CAD build for the part. Positions are in the model's coordinates, mm. A direction names the side the tool comes from. Coordinates: 2 decimals unless noted, no trailing zeros. Write each loop counter-clockwise with the first axis right and the second up, starting at its lowest first coordinate (ties: lowest second). Pieces come first, ordered by that corner, then holes. Notation, with made-up numbers: (-23, -11.5) -> (0, -11.5) arc R21 ccw to (0, -2.5) -> close; hole circle Ø6 at (42, 80.5). An arc over 180 degrees is marked (long way). Answer as CSV lines item,"result".
```python
from build123d import *

# Parameters (mm, degrees)
BOSS_EXTRUDE1_DEPTH = 7.75
SKETCH2_R           = 6.125
CUT_EXTRUDE1_DEPTH  = 4.25
CUT_EXTRUDE2_REACH  = 5.5
SKETCH3_R           = 2.125
SKETCH4_R           = 11
BOSS_EXTRUDE2_DEPTH = 20
SKETCH5_R           = 2.25
SKETCH5_R_2         = 4
CUT_EXTRUDE3_DEPTH  = 10
SKETCH6_R           = 2.125
CUT_EXTRUDE4_DEPTH  = 28.75
SKETCH10_R          = 2.75
CUT_EXTRUDE5_DEPTH  = 6


with BuildPart() as part:
    # Sketch1 → Boss-Extrude1 (new body)
    with BuildSketch(Plane.XY):
        with BuildLine():
            ThreePointArc((-12.5, 0), (0, -12.5), (12.5, 0))
            add(Edge.make_bspline(
                [(7.5, 49.5), (7.5, 26.668276539), (12.5, 15.631461909), (12.5, 0)],
                knots=[0, 0, 0, 0, 1, 1, 1, 1], degree=3))
            ThreePointArc((7.5, 49.5), (0, 57), (-7.5, 49.5))
            add(Edge.make_bspline(
                [(-7.5, 49.5), (-7.5, 26.668276539), (-12.5, 15.631461909), (-12.5, 0)],
                knots=[0, 0, 0, 0, 1, 1, 1, 1], degree=3))
        make_face()
    extrude(amount=BOSS_EXTRUDE1_DEPTH)

    # Sketch2 → Cut-Extrude1 (cut)
    with BuildSketch(Plane.XY.offset(7.75)):
        with Locations((0, 49.5)):
            Circle(SKETCH2_R)
    extrude(amount=-CUT_EXTRUDE1_DEPTH, mode=Mode.SUBTRACT)

    # Sketch3 → Cut-Extrude2 (cut, up to next)
    with BuildSketch(Plane.XY.offset(3.5), mode=Mode.PRIVATE) as cut_extrude2_sk1:
        with Locations((0, 49.5)):
            Circle(SKETCH3_R)
    cut_extrude2_tool1 = extrude(cut_extrude2_sk1.sketch, amount=-CUT_EXTRUDE2_REACH, mode=Mode.PRIVATE) & part.part
    add(cut_extrude2_tool1.solids().sort_by_distance((0, 49.5, 3.5))[0], mode=Mode.SUBTRACT)

    # Sketch4 → Boss-Extrude2 (add)
    with BuildSketch(Plane.XY.offset(7.75)):
        Circle(SKETCH4_R)
    extrude(amount=BOSS_EXTRUDE2_DEPTH)

    # Sketch5 → Cut-Extrude3 (cut)
    with BuildSketch(Plane.XY.offset(27.75)):
        with Locations((5.303300859, 5.303300859)):
            Circle(SKETCH5_R)
        with Locations((5.303300859, -5.303300859)):
            Circle(SKETCH5_R)
        with Locations((-5.303300859, -5.303300859)):
            Circle(SKETCH5_R)
        with Locations((-5.303300859, 5.303300859)):
            Circle(SKETCH5_R)
        Circle(SKETCH5_R_2)
    extrude(amount=-CUT_EXTRUDE3_DEPTH, mode=Mode.SUBTRACT)

    # Sketch6 → Cut-Extrude4 (cut, through all)
    with BuildSketch(Plane(origin=(0, 0, 0), x_dir=(-1, 0, 0), z_dir=(0, 0, -1))):
        Circle(SKETCH6_R)
    extrude(amount=-CUT_EXTRUDE4_DEPTH, mode=Mode.SUBTRACT)

    # Sketch10 → Cut-Extrude5 (cut)
    with BuildSketch(Plane(origin=(0, 0, 0), x_dir=(-1, 0, 0), z_dir=(0, 0, -1))):
        Circle(SKETCH10_R)
    extrude(amount=-CUT_EXTRUDE5_DEPTH, mode=Mode.SUBTRACT)


solid = part.part
```
Item 1: Wall check: line 1 (Y direction, x = 0, z = 2.1) (3 decimals); line 2 (Y direction, x = 0, z = 25); line 3 (X direction, y = -5, z = 19). Give the ranges that are in metal, low to high. Write a range as from..to.
Answer below:
line 1,"y = -12.5..-2.75, 2.75..47.375, 51.625..57"
line 2,"y = -11..-4, 4..11"
line 3,"x = -9.8..-7.53, -3.07..3.07, 7.53..9.8"
Item 2: Saw through at A-A on x = 0. Give the cut face in (y, z) (3 decimals), and give its area (3 significant figures).
Answer below:
outline,"(-12.5, 0) -> (-2.75, 0) -> (-2.75, 6) -> (-2.125, 6) -> (-2.125, 17.75) -> (-4, 17.75) -> (-4, 27.75) -> (-11, 27.75) -> (-11, 7.75) -> (-12.5, 7.75) -> close; (2.125, 6) -> (2.75, 6) -> (2.75, 0) -> (47.375, 0) -> (47.375, 3.5) -> (43.375, 3.5) -> (43.375, 7.75) -> (11, 7.75) -> (11, 27.75) -> (4, 27.75) -> (4, 17.75) -> (2.125, 17.75) -> close; (51.625, 0) -> (57, 0) -> (57, 7.75) -> (55.625, 7.75) -> (55.625, 3.5) -> (51.625, 3.5) -> close"
area,"749 mm2"
Item 3: Saw through at B-B on z = 9.75. Give the cut face in (x, y) (3 decimals), and give its area (3 significant figures).
Answer below:
outline,"circle Ø22 at (0, 0); hole circle Ø4.25 at (0, 0)"
area,"366 mm2"
Item 4: Flat gauge pins, fed straight in: pin 1 (2.5 mm diameter, centred on x = 5.3, y = -5.3, fed in from +Z); pin 2 (3 mm diameter, centred on y = 1.5, z = 20.5, fed in from +X); pin 3 (8 mm diameter, centred on y = 32, z = 6, fed in from +X). Where does each tip first touch, or does it go through?
Answer below:
pin 1,"stops at z = 17.75"
pin 2,"stops at x = 11"
pin 3,"stops at x = 9.07"
Item 5: Saw through at C-C on z = 25.5. Give the cut face in (x, y).
Answer below:
outline,"circle Ø22 at (0, 0); hole circle Ø4.5 at (-5.3, -5.3); hole circle Ø4.5 at (-5.3, 5.3); hole circle Ø8 at (0, 0); hole circle Ø4.5 at (5.3, -5.3); hole circle Ø4.5 at (5.3, 5.3)"
Item 6: 3-axis set-ups, long thin cutter, end or side, ignore diameter. For faces 4 (the cylindrical face through (0.981, 47.615, 1.774)), 5 (the cylindrical face through (0.596, -2.685, 2.958)), 6 (the flat face through (5, 5, 17.75)): which of +Z, -Z, +X, -X, +Y, -Y reach the whole face in a straight line?
Answer below:
face 4,"+Z, -Z"
face 5,"-Z"
face 6,"+Z"
Item 7: Two-plate mould, pull along Y, no slides. Class faces 1 (the cylindrical face through (-2.38, -10.74, 17.61)), 2 (the flat face through (0, 23, 7.75)), 3 (the cylindrical face through (-7.09, -6.67, 22.82)): pulls with the +Y half, pulls with the -Y half, needs draft (parallel to the pull), parting line crosses it, or undercut.
Answer below:
face 1,"parting line crosses it"
face 2,"needs draft"
face 3,"undercut"
Item 8: Saw through at D-D on z = 2.5. State how many separate pieces and enclosed holes the cut face has, and give its area (3 significant figures).
Answer below:
separate pieces,"1"
enclosed holes,"2"
area,"1,260 mm2"
